Can you work these out from the model? Positions are in its coordinate system, mm. Give positions to 0.01 mm unless a question says otherwise; leave off trailing zeros. Order: outer loops, then holes, each group sorted by start corner. A loop starts at its lowest first (then second) coordinate and runs counter-clockwise, first axis right, second up. Notation, with made-up numbers: M -7.75,63 L 0.25,63 A28 cw 0.25,98 Z; hole C -33,47 d11. An arc over 180 degrees is marked long. Use one line per item in the form item = value. Start each with the question number.
1. I want a section at A-A, the plane z = -4.5. List the corners of the cut face in (x, y) for me.
2. Will these pins go through, and if not, where does the flat tip stop? P1, Ø3, axis at x = 12.5, z = -3.5, coming from the -Y side; P2, Ø1, axis at y = -8.5, z = -7.5, coming from the -X side; P3, Ø2, axis at x = 7, z = -8.5, coming from the -Y side.
3. I need wall thicknesses on L1, parallel to Y at x = -12, z = -7; L2, parallel to Y at x = -14, z = -7.5; L3, parallel to X at y = 15.5, z = -4.25. Which ranges of each line are inside material? Lowest first, please.
4. I want a section at B-B, the plane y = 1. List the corners of the cut face in (x, z) for me.
5. I want a section at C-C, the plane x = -21. List the corners of the cut face in (y, z) for me, and give its area (3 significant figures).
```python
from build123d import *

# Parameters (mm, degrees)
F1_DEPTH = 10


with BuildPart() as f1:
    # F0 (on Top) → F1 (new body)
    with BuildSketch(Plane.XY):
        Polygon((24.997267, 0.369631), (12.178524, 21.833084), (-12.818743, 21.463453), (-24.997267, -0.369631), (-12.178524, -21.833084), (12.818743, -21.463453), align=None)
    extrude(amount=-F1_DEPTH)


solid = f1.part
```
Check result:
q1.outline = M -25,-0.37 L -12.18,-21.83 L 12.82,-21.46 L 25,0.37 L 12.18,21.83 L -12.82,21.46 Z
q2.P1 = -21.49
q2.P2 = -20.44
q2.P3 = -21.56
q3.L1 = -21.83 to 21.48
q3.L2 = -18.78 to 19.35
q3.L3 = -16.15 to 15.96
q4.outline = M -24.23,-10 L 24.62,-10 L 24.62,0 L -24.23,0 Z
q5.outline = M -7.06,-10 L 6.8,-10 L 6.8,0 L -7.06,0 Z
q5.area = 139 mm2
